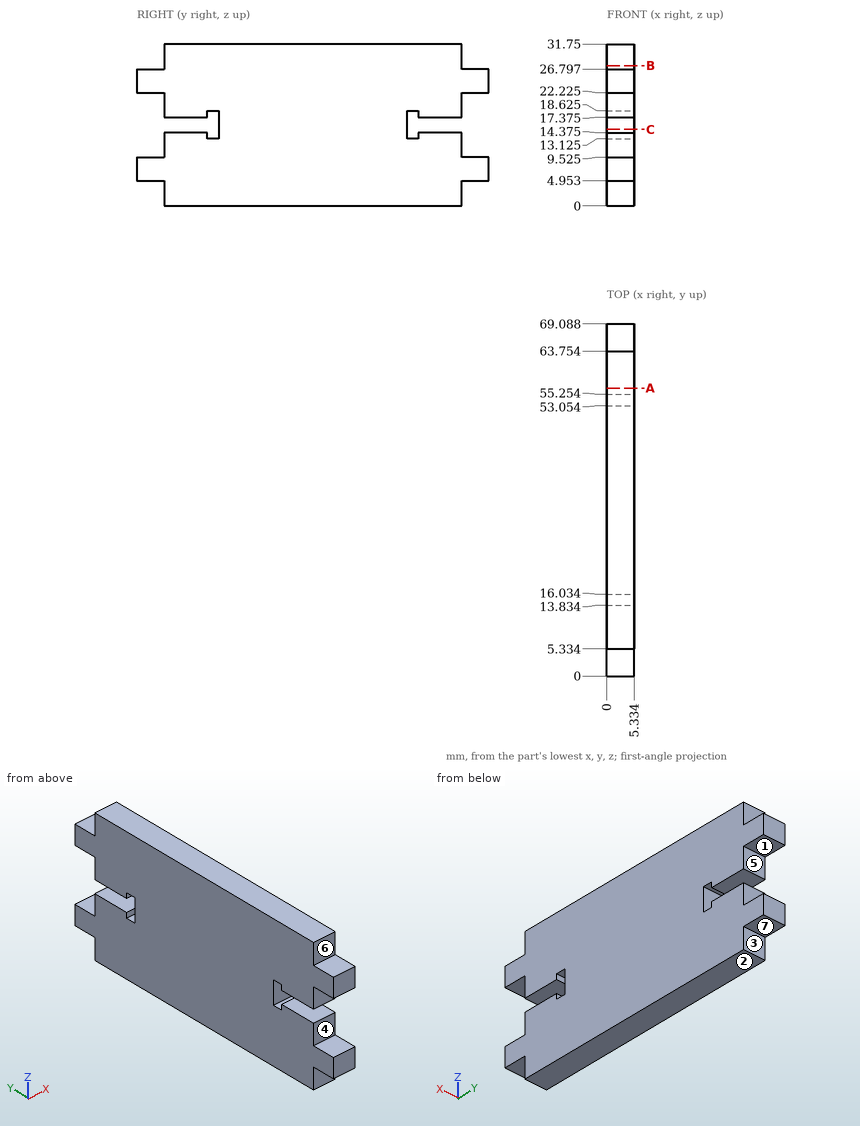
Geometry check sheet. Reference: drawing and pictorial views, mm from the part's lowest x, y, z. A direction names the side the tool comes from. Round coordinates to 2 decimals unless told otherwise and drop trailing zeros. Order: outer loops, then holes, each group sorted by start corner. A loop starts at its lowest first (then second) coordinate and runs counter-clockwise, first axis right, second up. Notation, with made-up numbers: (89, 72) - (121, 72) arc R28 cw to (121, 100) - close; hole circle Ø4 at (48, 17). An arc over 180 degrees is marked (long way). One line per question, with ' | ' between items. Start each with the question number.
(1) Sectioned sample at A-A on y = 56.5. Record the cut outline in (x, z) (3 decimals).
(2) Access from +Z, -Z, +X, -X, +Y, -Y to the whole of each face (thin tool, end or side, straight path). Record for the marked faces 4, 5, 6 and 7.
(3) Depth check by flat-ended pin: pin 1 Ø2.5 at (x, y) = (3, 14.5) entering from -Z; pin 2 Ø2.5 at (x, z) = (4, 16.5) entering from -Y; pin 3 Ø1.6 at (x, y) = (1.5, 66.5) entering from -Z; pin 4 Ø1 at (x, z) = (2.5, 3.5) entering from +Y. Enter the tip coordinate at first touch or a pass-through.
(4) Release check for a two-part mould opening along Z. For the marked faces 1, 2 and 3 record: released by +Z, released by -Z, zero draft, split by the parting line, or undercut.
(5) Sectioned sample at B-B on z = 27.5. Record the cut outline in (x, y), and give its area (3 significant figures).
(6) Sectioned sample at C-C on z = 15. Record the cut outline in (x, y).
(7) Thickness scan on L1, parallel to Y at x = 3.05, z = 18.5; L2, parallel to Z at x = 0.2, y = 59.5 (3 decimals); L3, parallel to Z at x = 0.9, y = 3 (3 decimals). Record the ranges inside material, lowest first. Write a range as [from, to].
Conclusion:
1) outline: (0, 0) - (5.334, 0) - (5.334, 14.375) - (0, 14.375) - close; (0, 17.375) - (5.334, 17.375) - (5.334, 31.75) - (0, 31.75) - close
2) face 4: +X, -X, -Y | face 5: +X, -X, +Y | face 6: +Z, +X, -X, -Y | face 7: -Z, +X, -X, +Y
3) pin 1: stops at z = 0 | pin 2: stops at y = 5.33 | pin 3: stops at z = 4.95 | pin 4: stops at y = 63.75
4) face 1: undercut | face 2: released by -Z | face 3: zero draft
5) outline: (0, 5.33) - (5.33, 5.33) - (5.33, 63.75) - (0, 63.75) - close | area: 312 mm2
6) outline: (0, 16.03) - (5.33, 16.03) - (5.33, 53.05) - (0, 53.05) - close
7) L1: y = [5.33, 13.83], [16.03, 53.05], [55.25, 63.75] | L2: z = [0, 14.375], [17.375, 31.75] | L3: z = [4.953, 9.525], [22.225, 26.797]
